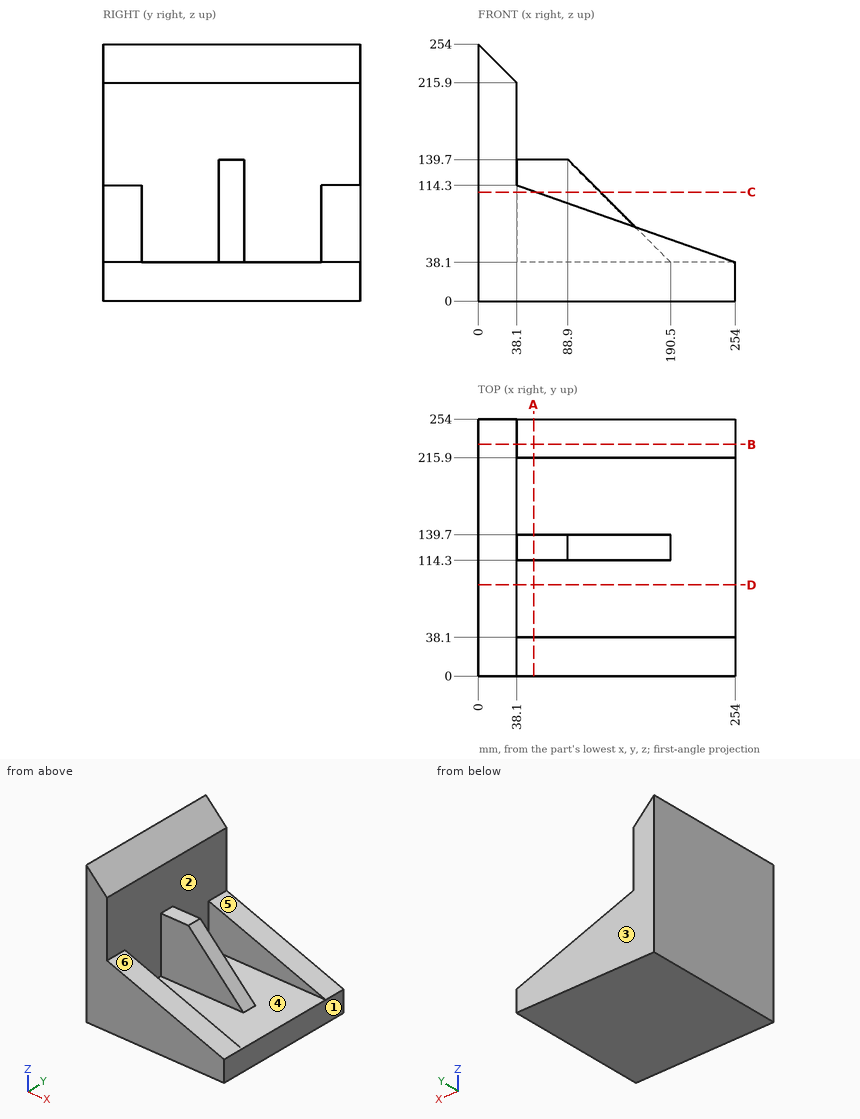
Study the drawing (mm; zero at the part's minimum x, y, z) and answer. A direction names the side the tool comes from. Round coordinates to 2 decimals unless told otherwise and drop trailing zeros. Write each loop counter-clockwise with the first axis right and the second up, starting at its lowest first coordinate (ties: lowest second). Pieces come first, ordered by that corner, then holes. Notation, with made-up numbers: (-32, 64) - (4, 64) arc R30 ccw to (4, 103) - close; hole circle Ø3 at (34.25, -9). An arc over 180 degrees is marked (long way). Use a Markdown table: item, result. Add a question column.
1. For a pull along Y with two mould halves and no side action, classify the marked faces 1, 2 and 3 as +Y half, -Y half, draft (parallel to the pull), parting line (faces both ways), or undercut.
2. Flat-ended cylindrical pins translate along their axes: P1, Ø8, axis at x = 208.5, y = 149, coming from the +Z side; P2, Ø10, axis at x = 182.5, y = 31.5, coming from the +Z side; P3, Ø2, axis at y = 79.5, z = 119, coming from the +X side. Find the tip coordinate at first contact, or state that the pin passes through.
3. The part is cut by section A-A (x = 55). Write down the section's boundary in (y, z), and give its area (3 significant figures).
4. The part is cut by section D-D (y = 90). Write down the section's boundary in (x, z), and give its area (3 significant figures).
5. The part is cut by section C-C (z = 107.5). Write down the section's boundary in (x, y), and give its area (3 significant figures).
6. Consider line 1 (Y direction, x = 112, z = 58); line 2 (Z direction, x = 186, y = 193). Determine where each line is inside the solid, lowest interval first.
7. The part is cut by section B-B (y = 229). Write down the section's boundary in (x, z), and give its area (3 significant figures).
8. A tool of negligible diameter and unlimited length cuts with its end or side. For the marked faces 4, 5 and 6, from which of +Z, -Z, +X, -X, +Y, -Y can it reach the whole face along a straight path? Write none if from no direction.
Reported:
| question | item | result |
|---|---|---|
| 1 | face 1 | draft |
| 1 | face 2 | undercut |
| 1 | face 3 | +Y half |
| 2 | P1 | z = 38.1 |
| 2 | P2 | z = 65.1 |
| 2 | P3 | x = 38.1 |
| 3 | outline | (0, 0) - (254, 0) - (254, 108.34) - (215.9, 108.34) - (215.9, 38.1) - (139.7, 38.1) - (139.7, 139.7) - (114.3, 139.7) - (114.3, 38.1) - (38.1, 38.1) - (38.1, 108.34) - (0, 108.34) - close |
| 3 | area | 17,600 mm^2 |
| 4 | outline | (0, 0) - (254, 0) - (254, 38.1) - (38.1, 38.1) - (38.1, 215.9) - (0, 254) - close |
| 4 | area | 17,200 mm^2 |
| 5 | outline | (0, 0) - (57.37, 0) - (57.37, 38.1) - (38.1, 38.1) - (38.1, 114.3) - (121.1, 114.3) - (121.1, 139.7) - (38.1, 139.7) - (38.1, 215.9) - (57.37, 215.9) - (57.37, 254) - (0, 254) - close |
| 5 | area | 13,300 mm^2 |
| 6 | line 1 | 0 to 38.1, 114.3 to 139.7, 215.9 to 254 |
| 6 | line 2 | 0 to 38.1 |
| 7 | outline | (0, 0) - (254, 0) - (254, 38.1) - (38.1, 114.3) - (38.1, 215.9) - (0, 254) - close |
| 7 | area | 25,400 mm^2 |
| 8 | face 4 | +Z, +X |
| 8 | face 5 | +Z, +X, +Y |
| 8 | face 6 | +Z, +X, -Y |
